The model under review builds one solid part; all positions refer to its coordinate system, in mm. Face numbers are marked on the shaded views. A direction names the side the tool comes from. Round coordinates to 2 decimals unless told otherwise and drop trailing zeros. Write each loop counter-clockwise with the first axis right and the second up, starting at its lowest first coordinate (ties: lowest second). Pieces come first, ordered by that corner, then holes. Notation, with made-up numbers: M -34,-10.75 L -9,-10.75 A27 ccw -9,9.25 Z; hole C 12,51 d9. An arc over 180 degrees is marked long. Write item = value, one per line. Start each with the question number.
Item 1: Take a section at C-C, the plane x = 0. Give the boundary of the cut face in (y, z), plus the area to 3 significant figures.
Item 2: For pin 1 Ø1 at (x, y) = (-43, 18) entering from -Z; pin 2 Ø3 at (x, y) = (57.5, -2.5) entering from -Z; pin 3 Ø3.5 at (x, y) = (70, -20) entering from +Z, all flat-tipped, find the tip position at first contact; note any pin that passes through.
Item 3: Tool access review of the marked faces 4 and 5: name each direction out of +Z, -Z, +X, -X, +Y, -Y from which nothing blocks a thin tool from reaching the whole face with its end or side.
Item 4: Take a section at D-D, the plane z = 310.75. Give the boundary of the cut face in (x, y), plus the area to 3 significant figures.
Item 5: To check wall thickness, follow line 1 along X through (y, z) = (20, 323.25); line 2 along Y through (x, z) = (70, 320.5); line 3 along Y through (x, z) = (-16, 328.75). State the ranges of each line that lie inside material, in increasing order.
Item 6: The part is to be moulded in two halves that separate along Y. For the marked faces 1, 2 and 3, say which applies: +Y half, -Y half, draft (parallel to the pull), parting line (faces both ways), or undercut.
Item 7: Take a section at A-A, the plane z = 324. Give the boundary of the cut face in (x, y).
Item 8: Take a section at B-B, the plane y = -15.5. Give the boundary of the cut face in (x, z).
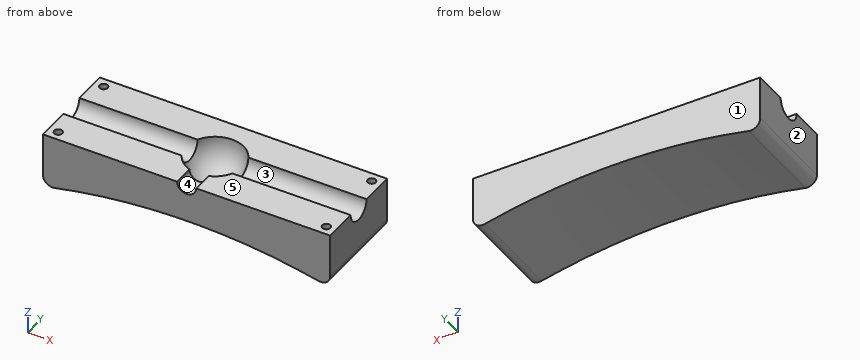
from build123d import *

# Parameters (mm, degrees)
F1_DEPTH = 25
F5_D     = 4.2
F5_DEPTH = 20
F5_TIP   = 1.2618073
F6_R     = 5


with BuildPart() as f1:
    # F0 (on Front) → F1 (new body, symmetric)
    with BuildSketch(Plane.XZ):
        with BuildLine():
            ThreePointArc((0, 315), (37.7725508345, 312.7270925319), (75, 305.9411708156))
            Line((75, 305.9411708156), (75, 335))
            Line((75, 335), (0, 335))
            Line((0, 335), (0, 315))
        make_face()
        with BuildLine():
            ThreePointArc((-75, 305.9411708156), (-37.7725508345, 312.7270925319), (0, 315))
            Line((0, 315), (0, 335))
            Line((0, 335), (-75, 335))
            Line((-75, 335), (-75, 305.9411708156))
        make_face()
    extrude(amount=F1_DEPTH, both=True)

    # F2 (on face) → F3 (revolve, cut)
    with BuildSketch(Plane.XY.offset(335)):
        with BuildLine():
            Line((-13.2664991614, 7), (-75, 7))
            Line((-75, 7), (-75, 0))
            Line((-75, 0), (-15, 0))
            ThreePointArc((-15, 0), (-14.5601766373, 3.6057254872), (-13.2664991614, 7))
        make_face()
        with BuildLine():
            ThreePointArc((13.2664991614, 7), (0, 15), (-13.2664991614, 7))
            ThreePointArc((-13.2664991614, 7), (-14.5601766373, 3.6057254872), (-15, 0))
            Line((-15, 0), (-13.2664991614, 0))
            Line((-13.2664991614, 0), (13.2664991614, 0))
            Line((13.2664991614, 0), (15, 0))
            ThreePointArc((15, 0), (14.5601766373, 3.6057254872), (13.2664991614, 7))
        make_face()
        with BuildLine():
            Line((75, 7), (13.2664991614, 7))
            ThreePointArc((13.2664991614, 7), (14.5601766373, 3.6057254872), (15, 0))
            Line((15, 0), (75, 0))
            Line((75, 0), (75, 7))
        make_face()
    revolve(axis=Axis((-44.1332495807, 0, 335), (1, 0, 0)), mode=Mode.SUBTRACT)

    # F5
    with Locations(Plane.XY.offset(335)):
        with Locations((-70, 20), (-70, -20), (70, 20), (70, -20)):
            Hole(F5_D / 2, depth=F5_DEPTH)
            with Locations((0, 0, -(F5_DEPTH + F5_TIP / 2))):  # 118° drill point
                Cone(0, F5_D / 2, F5_TIP, mode=Mode.SUBTRACT)

    # F6
    f6_edges = [f1.edges().sort_by_distance(p)[0] for p in [
        (-75, 0, 305.941171),
        (75, 0, 305.941171),
    ]]
    fillet(f6_edges, radius=F6_R)

    # F7 (on face) → F8 (revolve, cut)
    with BuildSketch(Plane.XY.offset(335)):
        with BuildLine():
            Line((0, 0), (-5, 0))
            Line((-5, 0), (-5, -14.1421356237))
            ThreePointArc((-5, -14.1421356237), (-2.5365296809, -14.7839783948), (0, -15))
            Line((0, -15), (0, 0))
        make_face()
        with BuildLine():
            ThreePointArc((0, -15), (-2.5365296809, -14.7839783948), (-5, -14.1421356237))
            Line((-5, -14.1421356237), (-5, -25))
            Line((-5, -25), (0, -25))
            Line((0, -25), (0, -15))
        make_face()
    revolve(axis=Axis((0, -12.5, 335), (0, -1, 0)), mode=Mode.SUBTRACT)


solid = f1.part
Response values:
q1.outline = M -25,315 L 25,315 L 25,335 L 15,335 A15 cw -14.14,330 L -25,330 Z
q1.area = 595 mm2
q2.pin_1 = 311.98
q2.pin_2 = 309.43
q2.pin_3 = 314.79
q3.face_4 = +Z, -Y
q3.face_5 = +Z, +X, -X, +Y, -Y
q4.outline = M -74.77,-25 L -51.57,-25 L -51.57,25 L -74.77,25 Z; M 51.57,-25 L 74.77,-25 L 74.77,25 L 51.57,25 Z
q4.area = 2,320 mm2
q5.line_1 = -75 to -72.1, -67.9 to 67.9, 72.1 to 75
q5.line_2 = -25 to -22.1, -17.9 to 17.9, 22.1 to 25
q5.line_3 = -25 to -3.15, 3.15 to 25
q6.face_1 = +Y half
q6.face_2 = draft
q6.face_3 = undercut
q7.outline = M -75,-25 L 75,-25 L 75,25 L -75,25 Z; hole C -70,-20 d4.2; hole C -70,20 d4.2; hole C 0,0 d20.4; hole C 70,-20 d4.2; hole C 70,20 d4.2
q8.outline = M -75,312.25 A5 ccw -68.91,307.37 A315 cw 68.91,307.37 A5 ccw 75,312.25 L 75,335 L 5,335 A5 cw -5,335 L -75,335 Z
